The listing builds one solid part. Answer for the finished solid, in the listing's coordinates (mm). Coordinates: 2 decimals unless noted, no trailing zeros. Order: outer loops, then holes, each group sorted by start corner. A loop starts at its lowest first (then second) coordinate and runs counter-clockwise, first axis right, second up. Notation, with made-up numbers: (31.25, -25.5) - (36.25, -25.5) arc R30 cw to (36.25, -0.5) - close; hole circle Ø6 at (66.5, -9). An arc over 180 degrees is marked (long way). Use one line per item in the form item = value. Start each with the question number.
Item 1: Consider line 1 along Y through (x, z) = (1.75, -7); line 2 along Y through (x, z) = (1.4, 11); line 3 along Y through (x, z) = (2.5, -37.5). Determine where each line is inside the solid, lowest interval first. Write a range as [from, to].
Item 2: Section C-C, the plane z = -51.2 is taken. Write down the section's boundary in (x, y), and give its area (3 significant figures).
Item 3: Each of these flat-tipped pins is pushed along its axis until it touches: pin 1 Ø1 at (x, z) = (1, 44) entering from -Y; pin 2 Ø0.5 at (x, y) = (1.5, -2) entering from +Z; pin 3 Ø1.6 at (x, z) = (1.5, -65.5) entering from +Y. Where does it stop, or does it pass through?
Item 4: The mould has two halves that part along Y. Classify faces 1 (the flat face through (3.18, -16, 1)), 2 (the cylindrical face through (1.568, -24.552, -27.505)): released by +Y, released by -Y, zero draft, split by the parting line, or undercut.
Item 5: Section A-A, the plane z = 19 is taken. Write down the section's boundary in (x, y).
Item 6: Section D-D, the plane z = -33 is taken. Write down the section's boundary in (x, y).
Item 7: Section B-B, the plane y = 46 is taken. Write down the section's boundary in (x, z), and give its area (3 significant figures).
from build123d import *

# Parameters (mm, degrees)
SKETCH1_W               = 152.4
SKETCH1_H               = 146.04
BOSS_EXTRUDE1_DEPTH     = 3.18
SKETCH3_R               = 1.4
SKETCH3_W               = 10
SKETCH3_H               = 3.18
BOSS_EXTRUDE5_DEPTH     = 3.18
CUT_EXTRUDE2_DEPTH      = 4.18
CUT_EXTRUDE3_DEPTH      = 4.18
SKETCH6_W               = 73
SKETCH6_H               = 26
CUT_EXTRUDE4_DEPTH      = 10
SKETCH7_R               = 1.47
CUT_EXTRUDE5_DEPTH      = 4.18
SKETCH8_R               = 4
CUT_EXTRUDE6_DEPTH      = 4.18
SKETCH9_W               = 47
SKETCH9_H               = 7
CUT_EXTRUDE7_DEPTH      = 1
CUT_EXTRUDE7_DEPTH_BACK = 4.18
SKETCH10_W              = 1.31
SKETCH10_H              = 2.5
CUT_EXTRUDE8_DEPTH      = 4.18
SKETCH11_R              = 1.4
CUT_EXTRUDE9_DEPTH      = 4.18


with BuildPart() as part:
    # Sketch1 → Boss-Extrude1 (new body)
    with BuildSketch(Plane(origin=(0, 0, 0), x_dir=(0, 0, -1), z_dir=(1, 0, 0))):
        Rectangle(SKETCH1_W, SKETCH1_H)
    extrude(amount=BOSS_EXTRUDE1_DEPTH)

    # Sketch3 → Boss-Extrude5 (add)
    with BuildSketch(Plane.ZY):
        Polygon((0, 73.02), (5, 73.02), (5, 76.2), (-5, 76.2), (-5, 73.02), align=None)
        with Locations((0, 74.61)):
            Circle(SKETCH3_R, mode=Mode.SUBTRACT)
        with Locations((0, -74.61)):
            Rectangle(SKETCH3_W, SKETCH3_H)
        with Locations((0, -74.61)):
            Circle(SKETCH3_R, mode=Mode.SUBTRACT)
    extrude(amount=-BOSS_EXTRUDE5_DEPTH)

    # Sketch4 → Cut-Extrude2 (cut, through all)
    with BuildSketch(Plane(origin=(0, 0, 0), x_dir=(0, 0, -1), z_dir=(1, 0, 0))):
        Polygon((-76.2, -5), (-76.2, 5), (-73.02, 5), (-73.02, 1.47), (-70.02, 1.47), (-70.02, 3.25), (-67.42, 3.25), (-67.42, 1.47), (-63.2, 1.47), (-63.2, -1.47), (-67.42, -1.47), (-67.42, -3.25), (-70.02, -3.25), (-70.02, -1.47), (-73.02, -1.47), (-73.02, -5), align=None)
    extrude(amount=CUT_EXTRUDE2_DEPTH, mode=Mode.SUBTRACT)

    # Sketch5 → Cut-Extrude3 (cut, through all)
    with BuildSketch(Plane.ZY):
        Polygon((-70.02, -1.47), (-73.02, -1.47), (-73.02, -5), (-76.2, -5), (-76.2, 5), (-73.02, 5), (-73.02, 1.47), (-70.02, 1.47), (-70.02, 3.25), (-67.42, 3.25), (-67.42, 1.47), (-63.2, 1.47), (-63.2, -1.47), (-67.42, -1.47), (-67.42, -3.25), (-70.02, -3.25), align=None)
    extrude(amount=-CUT_EXTRUDE3_DEPTH, mode=Mode.SUBTRACT)

    # Sketch6 → Cut-Extrude4 (cut)
    with BuildSketch(Plane.ZY):
        with Locations((0, 44.02)):
            Rectangle(SKETCH6_W, SKETCH6_H)
    extrude(amount=-CUT_EXTRUDE4_DEPTH, mode=Mode.SUBTRACT)

    # Sketch7 → Cut-Extrude5 (cut, through all)
    with BuildSketch(Plane.ZY):
        with Locations((-37.5, 59.52)):
            Circle(SKETCH7_R)
        with Locations((-37.5, 28.52)):
            Circle(SKETCH7_R)
        with Locations((37.5, 59.52)):
            Circle(SKETCH7_R)
        with Locations((37.5, 28.52)):
            Circle(SKETCH7_R)
    extrude(amount=-CUT_EXTRUDE5_DEPTH, mode=Mode.SUBTRACT)

    # Sketch8 → Cut-Extrude6 (cut, through all)
    with BuildSketch(Plane.ZY):
        with Locations((-51.2, -23.02)):
            Circle(SKETCH8_R)
        with Locations((-31.2, -23.02)):
            Circle(SKETCH8_R)
        with Locations((36.2, -23.02)):
            Circle(SKETCH8_R)
    extrude(amount=-CUT_EXTRUDE6_DEPTH, mode=Mode.SUBTRACT)

    # Sketch9 → Cut-Extrude7 (cut, two sides)
    with BuildSketch(Plane.ZY) as cut_extrude7_sk:
        Rectangle(SKETCH9_W, SKETCH9_H)
    extrude(amount=CUT_EXTRUDE7_DEPTH, mode=Mode.SUBTRACT)
    extrude(cut_extrude7_sk.sketch, amount=-CUT_EXTRUDE7_DEPTH_BACK, mode=Mode.SUBTRACT)

    # Sketch10 → Cut-Extrude8 (cut, through all)
    with BuildSketch(Plane.ZY):
        with Locations((43.855, -23.02)):
            Rectangle(SKETCH10_W, SKETCH10_H)
    extrude(amount=-CUT_EXTRUDE8_DEPTH, mode=Mode.SUBTRACT)

    # Sketch11 → Cut-Extrude9 (cut, through all)
    with BuildSketch(Plane.ZY):
        with Locations((-11, 14.02)):
            Circle(SKETCH11_R)
        with Locations((11, 14.02)):
            Circle(SKETCH11_R)
    extrude(amount=-CUT_EXTRUDE9_DEPTH, mode=Mode.SUBTRACT)


solid = part.part
Response:
q1.line_1 = [-73.02, -3.5], [3.5, 31.02], [57.02, 73.02]
q1.line_2 = [-73.02, -3.5], [3.5, 12.62], [15.42, 31.02], [57.02, 73.02]
q1.line_3 = [-73.02, 27.05], [29.99, 58.05], [60.99, 73.02]
q2.outline = (0, -73.02) - (3.18, -73.02) - (3.18, -27.02) - (0, -27.02) - close; (0, -19.02) - (3.18, -19.02) - (3.18, 73.02) - (0, 73.02) - close
q2.area = 439 mm2
q3.pin_1 = -73.02
q3.pin_2 = 73.02
q3.pin_3 = 73.02
q4.face_1 = zero draft
q4.face_2 = undercut
q5.outline = (0, -73.02) - (3.18, -73.02) - (3.18, -3.5) - (0, -3.5) - close; (0, 3.5) - (3.18, 3.5) - (3.18, 31.02) - (0, 31.02) - close; (0, 57.02) - (3.18, 57.02) - (3.18, 73.02) - (0, 73.02) - close
q6.outline = (0, -73.02) - (3.18, -73.02) - (3.18, -26.59) - (0, -26.59) - close; (0, -19.45) - (3.18, -19.45) - (3.18, 31.02) - (0, 31.02) - close; (0, 57.02) - (3.18, 57.02) - (3.18, 73.02) - (0, 73.02) - close
q7.outline = (0, -76.2) - (3.18, -76.2) - (3.18, -36.5) - (0, -36.5) - close; (0, 36.5) - (3.18, 36.5) - (3.18, 76.2) - (0, 76.2) - close
q7.area = 252 mm2
